Verification items for the finished model (mm, model axes). A direction names the side the tool comes from. Give positions to 0.01 mm unless a question says otherwise; leave off trailing zeros. Write each loop counter-clockwise with the first axis right and the second up, starting at its lowest first coordinate (ties: lowest second). Pieces come first, ordered by that corner, then holes.
from build123d import *

# Parameters (mm, degrees)
F1_DEPTH = 127
F3_DEPTH = 254


with BuildPart() as f1:
    # F0 (on Right) → F1 (new body)
    with BuildSketch(Plane.YZ):
        with BuildLine():
            Line((-21.34454, 0), (0, 0))
            Line((0, 0), (209.8645, 462.936498))
            ThreePointArc((209.8645, 462.936498), (221.179593, 513.382616), (211.45127, 564.158614))
            Line((211.45127, 564.158614), (183.866499, 630.458851))
            Line((183.866499, 630.458851), (-324.133501, 630.458851))
            Line((-324.133501, 630.458851), (-435.125129, 372.189923))
            Line((-435.125129, 372.189923), (-21.34454, 0))
        make_face()
    extrude(amount=F1_DEPTH)

    # F2 (on face) → F3 (cut)
    with BuildSketch(Plane.YZ.offset(127)):
        Polygon((-76.997541, 472.424954), (-230.415642, 400.5723), (-92.960328, 211.070791), (29.763866, 337.927192), (-113.02951, 357.656449), align=None)
    extrude(amount=-F3_DEPTH, mode=Mode.SUBTRACT)


solid = f1.part
Item 1: Release check for a two-part mould opening along Z. For faces 3 (the face through (63, -11, 0)), 4 (the face through (62.611, 221.166, 512.654)), 5 (the face through (64.39, -162.65, 307.15)) record: released by +Z, released by -Z, zero draft, split by the parting line, or undercut.
Answer key:
face 3: released by -Z
face 4: split by the parting line
face 5: undercut
Item 2: Sectioned sample at C-C on y = -202.5. Record the cut outline in (x, z).
Answer key:
outline: (0, 162.95) - (127, 162.95) - (127, 362.09) - (0, 362.09) - close; (0, 413.65) - (127, 413.65) - (127, 630.46) - (0, 630.46) - close
Item 3: Set-up check for faces 1 (the face through (127, -39, 390)), 2 (the face through (64.389, -95.266, 414.237)): record each of +Z, -Z, +X, -X, +Y, -Y from which the full face is reachable in a straight line by a thin tool's end or side.
Answer key:
face 1: +Z, -Z, +X, +Y, -Y
face 2: +X, -X
Item 4: Sectioned sample at D-D on y = 46. Record the cut outline in (x, z).
Answer key:
outline: (0, 101.47) - (127, 101.47) - (127, 630.46) - (0, 630.46) - close
Item 5: Sectioned sample at B-B on z = 442. Record the cut outline in (x, y), then the cut area to 3 significant figures.
Answer key:
outline: (0, -405.12) - (127, -405.12) - (127, -141.96) - (0, -141.96) - close; (0, -86.55) - (127, -86.55) - (127, 200.37) - (0, 200.37) - close
area: 69,900 mm2
Item 6: Depth check by flat-ended pin: pin 1 (3 mm diameter, centred on x = 93, y = -330.5, fed in from +Z); pin 2 (4 mm diameter, centred on x = 78, z = 396.5, fed in from -Y); pin 3 (8 mm diameter, centred on x = 37, y = -325, fed in from -Z). Enter the tip coordinate at first touch or a pass-through.
Answer key:
pin 1: stops at z = 619.13
pin 2: stops at y = -425.54
pin 3: stops at z = 269.54
Item 7: Sectioned sample at A-A on x = 31. Record the cut outline in (y, z), then the cut area to 3 significant figures.
Answer key:
outline: (-435.13, 372.19) - (-21.34, 0) - (0, 0) - (209.86, 462.94) arc R127 ccw to (211.45, 564.16) - (183.87, 630.46) - (-324.13, 630.46) - close; hole (-230.42, 400.57) - (-92.96, 211.07) - (29.76, 337.93) - (-113.03, 357.66) - (-77, 472.42) - close
area: 241,000 mm2
Item 8: Scan lines: line 1 along Y through (x, z) = (20, 418); line 2 along Y through (x, z) = (33, 322.5); line 3 along Z through (x, y) = (104.5, -223). Record each from-to range of solid material in increasing order.
Answer key:
line 1: y = -415.44 to -193.2, -94.08 to 189.49
line 2: y = -379.88 to -173.79, 14.84 to 146.2
line 3: z = 181.39 to 390.35, 404.05 to 630.46
